For this review, take the finished solid that the model builds, in its own axes (mm). A direction names the side the tool comes from. Give positions to 0.01 mm unless a question says otherwise; leave off trailing zeros. Write each loop counter-clockwise with the first axis right and the second up, starting at its lowest first coordinate (ties: lowest second). Pieces come first, ordered by that corner, then holes.
1) We need section A-A on z = 12. Give the boundary of the cut face in (x, y), and give its area (3 significant figures).
2) Wall thickness on line 1 along Y through (x, z) = (-168, 32); line 2 along Y through (x, z) = (-109, 3); line 3 along X through (y, z) = (12, 27.5): over which ranges is each line inside the solid? List them lowest first.
3) Machinability: for faces 4 (the face through (-114, 48, -4)), 5 (the face through (3.549, 4.754, 34.498)), 6 (the face through (-6, 67.76, 35)), which of the approach directions +Z, -Z, +X, -X, +Y, -Y give a long, thin tool a straight path to every point of the face, cutting with its end or side? Answer none if there is none.
4) For P1, Ø1, axis at x = -47.5, y = 30.5, coming from the +Z side; P2, Ø3, axis at x = -3, y = 25.5, coming from the +Z side; P3, Ø6.5, axis at x = -166, y = 91, coming from the +Z side, all flat-tipped, find the tip position at first contact; note any pin that passes through.
5) Draft analysis for pull direction X (two halves, no side actions). For faces 1 (the face through (-81, 102, 35)), 2 (the face through (-232, 11, 35)), 3 (the face through (-133, 0, 35)), state which applies: pulls with the +X half, pulls with the -X half, needs draft (parallel to the pull), parting line crosses it, or undercut.
6) We need section B-B on y = 7.5. Give the boundary of the cut face in (x, z), and give its area (3 significant figures).
7) We need section C-C on x = -184. Give the boundary of the cut face in (y, z), and give its area (3 significant figures).
from build123d import *

# Parameters (mm, degrees)
F1_DEPTH = 72
F3_DEPTH = 4
F5_DEPTH = 4
F7_DEPTH = 25
F8_R     = 3
F9_DEPTH = 5.5


with BuildPart() as f1:
    # F0 (on Top) → F1 (new body)
    with BuildSketch(Plane.XY):
        Polygon((-232, 28.7712871801), (-232, 9), (-232, -7), (7, -7), (7, 102), (-170.6706311353, 102), align=None)
        with BuildLine():
            Line((0, 9), (0, 0))
            Line((0, 0), (-21.3304098297, 0))
            ThreePointArc((-21.3304098297, 0), (-22.567460882, -0.0826411216), (-23.8045119343, 0))
            Line((-23.8045119343, 0), (-39.7422893838, 0))
            ThreePointArc((-39.7422893838, 0), (-41.1674409876, -0.1098453274), (-42.5925925915, 0))
            Line((-42.5925925915, 0), (-59.7671166301, 0))
            Line((-59.7671166301, 0), (-78.3671166301, 0))
            Line((-78.3671166301, 0), (-96.9671166301, 0))
            Line((-96.9671166301, 0), (-115.5671166301, 0))
            Line((-115.5671166301, 0), (-134.1671166301, 0))
            Line((-134.1671166301, 0), (-152.7671166301, 0))
            Line((-152.7671166301, 0), (-171.3671166301, 0))
            Line((-171.3671166301, 0), (-189.9671166301, 0))
            Line((-189.9671166301, 0), (-208.5671166301, 0))
            Line((-208.5671166301, 0), (-225, 0))
            Line((-225, 0), (-225, 9))
            Line((-225, 9), (-225, 19.009443))
            Line((-225, 19.009443), (-216.0657793283, 19.009443))
            Line((-216.0657793283, 19.009443), (-216.0657793283, 33.8660545808))
            Line((-216.0657793283, 33.8660545808), (-218.6024326595, 33.8660545808))
            Line((-218.6024326595, 33.8660545808), (-176.2169181556, 84.4753585209))
            Line((-176.2169181556, 84.4753585209), (-160.9487113722, 84.4753585209))
            Line((-160.9487113722, 84.4753585209), (-160.9487113722, 95))
            Line((-160.9487113722, 95), (0, 95))
            Line((0, 95), (0, 80.24520114))
            Line((0, 80.24520114), (-12.4263259421, 80.2028560212))
            Line((-12.4263259421, 80.2028560212), (-12.3839236644, 67.7597565904))
            Line((-12.3839236644, 67.7597565904), (0, 67.7597565904))
            Line((0, 67.7597565904), (0, 30.28925322))
            Line((0, 30.28925322), (-9.0186540037, 30.28925322))
            Line((-9.0186540037, 30.28925322), (-9.0186540037, 19.0464295447))
            Line((-9.0186540037, 19.0464295447), (0, 19.0464295447))
            Line((0, 19.0464295447), (0, 9))
        make_face(mode=Mode.SUBTRACT)
    extrude(amount=F1_DEPTH)

    # F2 (on Top) → F3 (join)
    with BuildSketch(Plane.XY):
        Polygon((-170.6706311353, 102), (-232, 28.7712871801), (-232, -7), (7, -7), (7, 102), align=None)
    extrude(amount=-F3_DEPTH)

    # F4 (on face) → F5 (join)
    with BuildSketch(Plane.XY.offset(72)):
        Polygon((7, 102), (-170.6706311353, 102), (-232, 28.7712871801), (-232, -7), (7, -7), align=None)
        Polygon((-230, -5), (-230, 28.0444074988), (-169.7368749983, 100), (5, 100), (5, -5), align=None, mode=Mode.SUBTRACT)
    extrude(amount=F5_DEPTH)

    # F6 (on face) → F7 (cut)
    with BuildSketch(Plane.YZ.offset(7)):
        with BuildLine():
            Line((4.5232147723, 36), (14.5232147723, 36))
            ThreePointArc((14.5232147723, 36), (9.5232147723, 41), (4.5232147723, 36))
        make_face()
        with BuildLine():
            ThreePointArc((4.5232147723, 36), (9.5232147723, 31), (14.5232147723, 36))
            Line((14.5232147723, 36), (4.5232147723, 36))
        make_face()
    extrude(amount=-F7_DEPTH, mode=Mode.SUBTRACT)

    # F8 (on face) → F9 (cut)
    with BuildSketch(Plane.XY.offset(72)):
        with Locations((-167.3095971346, 89.7376792604)):
            Circle(F8_R)
        with Locations((-222.2577780485, 26.4377487904)):
            Circle(F8_R)
        with Locations((-5.7860915549, 73.9813063058)):
            Circle(F8_R)
        with Locations((-3.1610322185, 24.6678413823)):
            Circle(F8_R)
    extrude(amount=-F9_DEPTH, mode=Mode.SUBTRACT)


solid = f1.part
Results list:
1. outline: (-232, -7) - (7, -7) - (7, 102) - (-170.67, 102) - (-232, 28.77) - close; hole (-225, 0) - (-42.59, 0) arc R9.3 ccw to (-39.74, 0) - (-23.8, 0) arc R9.3 ccw to (-21.33, 0) - (0, 0) - (0, 19.05) - (-9.02, 19.05) - (-9.02, 30.29) - (0, 30.29) - (0, 67.76) - (-12.38, 67.76) - (-12.43, 80.2) - (0, 80.25) - (0, 95) - (-160.95, 95) - (-160.95, 84.48) - (-176.22, 84.48) - (-218.6, 33.87) - (-216.07, 33.87) - (-216.07, 19.01) - (-225, 19.01) - close
1. area: 4,890 mm2
2. line 1: y = -7 to 0, 84.48 to 102
2. line 2: y = -7 to 0, 95 to 102
2. line 3: x = -232 to -225, 0 to 7
3. face 4: -Z, +X, -X, +Y, -Y
3. face 5: +X
3. face 6: +Z
4. P1: stops at z = 0
4. P2: stops at z = 66.5
4. P3: stops at z = 72
5. face 1: needs draft
5. face 2: pulls with the -X half
5. face 3: undercut
6. outline: (-232, -4) - (7, -4) - (7, 31.43) - (0, 31.43) - (0, 0) - (-225, 0) - (-225, 72) - (-230, 72) - (-230, 76) - (-232, 76) - close; (0, 40.57) - (7, 40.57) - (7, 76) - (5, 76) - (5, 72) - (0, 72) - close
6. area: 1,920 mm2
7. outline: (-7, -4) - (86.08, -4) - (86.08, 76) - (82.97, 76) - (82.97, 72) - (75.18, 72) - (75.18, 0) - (0, 0) - (0, 72) - (-5, 72) - (-5, 76) - (-7, 76) - close
7. area: 1,680 mm2
